Geometry: final body of the model. Coordinates: model frame, mm. A direction names the side the tool comes from. Give positions to 0.01 mm unless a question says otherwise; leave off trailing zeros. Write each loop counter-clockwise with the first axis right and the second up, starting at its lowest first coordinate (ties: lowest second). Pieces come first, ordered by that corner, then holes. Notation, with made-up numbers: M 25.5,-1.5 L 81.5,-1.5 A11 cw 81.5,8.5 Z; hole C 3.5,24 d3. An arc over 180 degrees is marked long. Answer as a JSON object with one key per item and string values.
from build123d import *

# Parameters (mm, degrees)
F0_W           = 37
F0_H           = 20
F1_DEPTH       = 10
F2_D           = 5.6
F2_CBORE_D     = 9.75
F2_CBORE_DEPTH = 5
F3_W           = 2.75
F3_H           = 20
F4_DEPTH       = 6
F5_SIZE        = 0.3


with BuildPart() as f1:
    # F0 (on Front) → F1 (new body)
    with BuildSketch(Plane.XZ):
        Rectangle(F0_W, F0_H)
    extrude(amount=-F1_DEPTH)

    # F2 (through all)
    with Locations(Plane.XZ):
        with Locations((6.5, 0)):
            CounterBoreHole(F2_D / 2, F2_CBORE_D / 2, F2_CBORE_DEPTH)

    # F3 (on face) → F4 (join)
    with BuildSketch(Plane(origin=(-18.5, 0, 0), x_dir=(0, -1, 0), z_dir=(-1, 0, 0))):
        with Locations((-3.125, 0)):
            Rectangle(F3_W, F3_H)
    extrude(amount=F4_DEPTH)

    # F5
    f5_edges = [f1.edges().sort_by_distance(p)[0] for p in [
        (0, 0, 10),
        (-18.5, 0, 0),
        (0, 0, -10),
        (18.5, 0, 0),
        (18.5, 5, -10),
        (18.5, 5, 10),
        (-18.5, 0.875, -10),
        (-18.5, 7.25, -10),
        (-24.5, 3.125, -10),
        (-24.5, 3.125, 10),
        (-18.5, 0.875, 10),
        (-18.5, 7.25, 10),
        (-24.5, 1.75, 0),
        (-24.5, 4.5, 0),
        (-18.5, 10, 0),
        (0, 10, 10),
        (0, 10, -10),
        (18.5, 10, 0),
        (1.625, 0, 0),
    ]]
    chamfer(f5_edges, length=F5_SIZE)


solid = f1.part
1) Cut plane B-B on z = 0. Return loops of the section in (x, y) (3 decimals).
Geometry check:
{"outline": "M -24.5,2.05 L -24.2,1.75 L -18.5,1.75 L -18.5,0.3 L -18.2,0 L 1.325,0 L 1.625,0.3 L 1.625,5 L 3.7,5 L 3.7,10 L -18.2,10 L -18.5,9.7 L -18.5,4.5 L -24.2,4.5 L -24.5,4.2 Z; M 9.3,5 L 11.375,5 L 11.375,0.3 L 11.675,0 L 18.2,0 L 18.5,0.3 L 18.5,9.7 L 18.2,10 L 9.3,10 Z"}
2) Set-up query: faces 1 (the flat face through (-18.5, 1, 0)), 2 (the flat face through (9, 5, -2)), 3 (the flat face through (0, 10, 0)). Return all of +Z, -Z, +X, -X, +Y, -Y with unobstructed straight access to the full face (end or side cutting, diameter ignored); none if empty.
Geometry check:
{"face 1": "+Z, -Z, -X, -Y", "face 2": "-Y", "face 3": "+Z, -Z, +X, -X, +Y"}
3) Contact query for flat-ended pins moving along their axis: P1, Ø6.5, axis at x = -21.5, z = 0.5, coming from the -Y side; P2, Ø4, axis at y = 7.5, z = 2.5, coming from the -X side; P3, Ø4, axis at x = 4.5, z = 1.5, coming from the -Y side. Output: stop coordinate, or through.
Geometry check:
{"P1": "stops at y = 0.05", "P2": "stops at x = -18.5", "P3": "stops at y = 5"}
4) Cut plane D-D on z = 6.25. Return loops of the section in (x, y).
Geometry check:
{"outline": "M -24.5,2.05 L -24.2,1.75 L -18.5,1.75 L -18.5,0.3 L -18.2,0 L 18.2,0 L 18.5,0.3 L 18.5,9.7 L 18.2,10 L -18.2,10 L -18.5,9.7 L -18.5,4.5 L -24.2,4.5 L -24.5,4.2 Z"}
5) Line query: line 1 (Z direction, x = 6.5, y = 3.95) (3 decimals); line 2 (Z direction, x = 6.5, y = 6.1); line 3 (X direction, y = 5.5, z = 4). Output: solid intervals per line, ascending. Write a range as from..to.
Geometry check:
{"line 1": "z = -10..-4.875, 4.875..10", "line 2": "z = -10..-2.8, 2.8..10", "line 3": "x = -18.5..18.5"}
6) Cut plane A-A on x = 6.5. Return loops of the section in (y, z) (3 decimals), and give its area (3 significant figures).
Geometry check:
{"outline": "M 0,-9.7 L 0.3,-10 L 9.7,-10 L 10,-9.7 L 10,-2.8 L 5,-2.8 L 5,-4.875 L 0.3,-4.875 L 0,-5.175 Z; M 0,5.175 L 0.3,4.875 L 5,4.875 L 5,2.8 L 10,2.8 L 10,9.7 L 9.7,10 L 0.3,10 L 0,9.7 Z", "area": "123 mm2"}
7) Cut plane C-C on y = 2.5. Return loops of the section in (x, z) (3 decimals), and give its area (3 significant figures).
Geometry check:
{"outline": "M -24.5,-9.7 L -24.2,-10 L 18.2,-10 L 18.5,-9.7 L 18.5,9.7 L 18.2,10 L -24.2,10 L -24.5,9.7 Z; hole C 6.5,0 d9.75", "area": "785 mm2"}
8) Pull-direction query (Z, two-part tool) for faces 4 (the cylindrical face through (3.83, 7.54, 0.84)), 5 (the flat face through (-18.5, 7, 0)), 6 (the flat face through (-3, 5, 10)), 7 (the flat face through (-3, 5, -10)); classes: pulls with the +Z half, pulls with the -Z half, needs draft (parallel to the pull), parting line crosses it, or undercut.
Geometry check:
{"face 4": "undercut", "face 5": "needs draft", "face 6": "pulls with the +Z half", "face 7": "pulls with the -Z half"}
